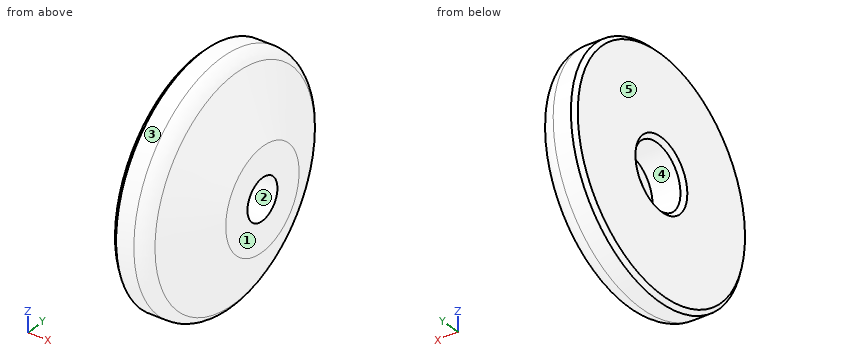
```python
from build123d import *

# Parameters (mm, degrees)
FILLET1_R     = 2
CHAMFER1_SIZE = 0.5


with BuildPart() as part:
    # Sketch1 → Revolve1 (revolve)
    with BuildSketch(Plane.XY, mode=Mode.PRIVATE) as revolve1_sk:
        Polygon((0, 4), (0, 15), (4, 15), (8, 6.362924355), (8, 2.6), (4, 2.6), (4, 4), align=None)
    revolve(revolve1_sk.sketch.rotate(Axis((0, 0, 0), (1, 0, 0)), 90), axis=Axis((0, 0, 0), (1, 0, 0)))

    # Fillet1
    fillet1_edges = [part.edges().sort_by_distance(p)[0] for p in [
        (4, 0, -15),
    ]]
    fillet(fillet1_edges, radius=FILLET1_R)

    # Chamfer1
    chamfer1_edges = [part.edges().sort_by_distance(p)[0] for p in [
        (0, 0, -15),
        (0, 0, -4),
    ]]
    chamfer(chamfer1_edges, length=CHAMFER1_SIZE)


solid = part.part
```
Input: part model. Units: mm. Frame: model coordinates. Face numbers are marked on the shaded views. A direction names the side the tool comes from. Give positions to 0.01 mm unless a question says otherwise; leave off trailing zeros. Loops run counter-clockwise (first coordinate to the right, second up) from the corner with the lowest first, then second, coordinate; pieces in that order, holes last. Notation, with made-up numbers: M 60.25,50.5 L 113.25,50.5 A20 cw 113.25,65.5 Z; hole C 79.25,-23 d2. An arc over 180 degrees is marked long. Answer as CSV lines item,"result". Start each with the question number.
1. Pin query (flat end, axial travel): P1, Ø1, axis at x = 2.5, z = 11.5, coming from the -Y side; P2, Ø2.5, axis at y = -1, z = 1.5, coming from the -X side; P3, Ø5, axis at y = 0, z = 0, coming from the -X side; P4, Ø2, axis at x = 2, z = 5.5, coming from the +Y side. Return the tip coordinate at first contact, or that it passes through.
2. Reachability of the marked faces 4 and 5 from +Z, -Z, +X, -X, +Y, -Y: full face, straight path, thin tool, end or side. Return the list, or none.
3. Section A-A on x = 5.25. Return loops of the section in (y, z), plus the area to 3 significant figures.
4. Section B-B on x = 1.25. Return loops of the section in (y, z).
5. Pull-direction query (Z, two-part tool) for the marked faces 1, 2 and 3; classes: released by +Z, released by -Z, zero draft, split by the parting line, or undercut.
6. Line query: L1, parallel to Y at x = 2.25, z = 0; L2, parallel to Y at x = 4.5, z = -1.5; L3, parallel to Z at x = 7, y = 0.5. Output: solid intervals per line, ascending.
Computed values:
1,P1,"stops at y = -10.2"
1,P2,"stops at x = 4"
1,P3,"passes through"
1,P4,"stops at y = 14.31"
2,face 4,"-X"
2,face 5,"+Z, -Z, -X, +Y, -Y"
3,outline,"C 0,0 d24.6; hole C 0,0 d5.2"
3,area,"454 mm²"
4,outline,"C 0,0 d30; hole C 0,0 d8"
5,face 1,"zero draft"
5,face 2,"undercut"
5,face 3,"split by the parting line"
6,L1,"y = -15 to -4, 4 to 15"
6,L2,"y = -13.84 to -2.12, 2.12 to 13.84"
6,L3,"z = -8.51 to -2.55, 2.55 to 8.51"
